Design review of the part shown in the three views and the two pictorial views. Dimensions are in mm from the part's minimum x, y and z. Give positions to 0.01 mm unless a question says otherwise; leave off trailing zeros. Loops run counter-clockwise (first coordinate to the right, second up) from the corner with the lowest first, then second, coordinate; pieces in that order, holes last. Notation, with made-up numbers: (33.25, -3) - (90.25, -3) arc R12 ccw to (90.25, 4) - close; hole circle Ø10 at (56.25, -3). An arc over 180 degrees is marked (long way). Answer as a JSON object with one key per item and string values.
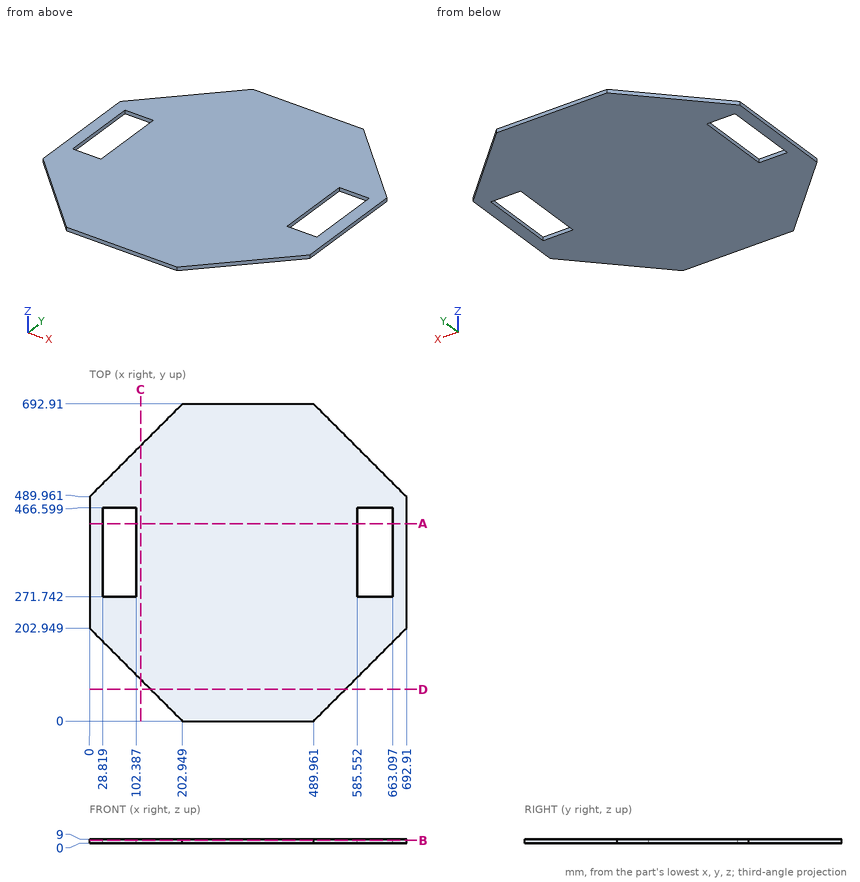
Q1. Clearance check with flat-ended pins moving along their axes: pin 1 Ø5 at (x, y) = (588.5, 261) entering from -Z; pin 2 Ø2.5 at (x, z) = (630, 5) entering from +Y; pin 3 Ø4.5 at (x, z) = (59, 5) entering from -Y; pin 4 Ø1.5 at (x, z) = (171.5, 6) entering from +Y. State where each tip first meets the part, or that it passes through.
Results:
{"pin 1": "stops at z = 0", "pin 2": "stops at y = 554.12", "pin 3": "stops at y = 141.7", "pin 4": "stops at y = 662.21"}
Q2. To check wall thickness, follow probe 1 along X at (y, z) = (437, 3.75); probe 2 along Y at (x, z) = (634, 3.25) (1 decimal); probe 3 along X at (y, z) = (643, 5.75). State the ranges of each line that lie inside material, in increasing order. Write a range as [from, to].
Results:
{"probe 1": "x = [0, 28.82], [102.39, 585.55], [663.1, 692.91]", "probe 2": "y = [144, 271.7], [466.6, 548.9]", "probe 3": "x = [153.04, 539.87]"}
Q3. Consider section D-D, the plane y = 69. State the section outline as (x, z) points.
Results:
{"outline": "(133.95, 0) - (558.96, 0) - (558.96, 9) - (133.95, 9) - close"}
Q4. Consider section C-C, the plane x = 112. State the section outline as (y, z) points.
Results:
{"outline": "(90.95, 0) - (601.96, 0) - (601.96, 9) - (90.95, 9) - close"}
Q5. Consider section B-B, the plane z = 6.25. State the section outline as (x, y) points, plus the area to 3 significant figures.
Results:
{"outline": "(0, 202.95) - (202.95, 0) - (489.96, 0) - (692.91, 202.95) - (692.91, 489.96) - (489.96, 692.91) - (202.95, 692.91) - (0, 489.96) - close; hole (28.82, 271.74) - (102.39, 271.74) - (102.39, 466.6) - (28.82, 466.6) - close; hole (585.55, 271.74) - (663.1, 271.74) - (663.1, 466.6) - (585.55, 466.6) - close", "area": "368,000 mm^2"}
Q6. Consider section A-A, the plane y = 431.5. State the section outline as (x, z) points, plus the area to 3 significant figures.
Results:
{"outline": "(0, 0) - (28.82, 0) - (28.82, 9) - (0, 9) - close; (102.39, 0) - (585.55, 0) - (585.55, 9) - (102.39, 9) - close; (663.1, 0) - (692.91, 0) - (692.91, 9) - (663.1, 9) - close", "area": "4,880 mm^2"}
